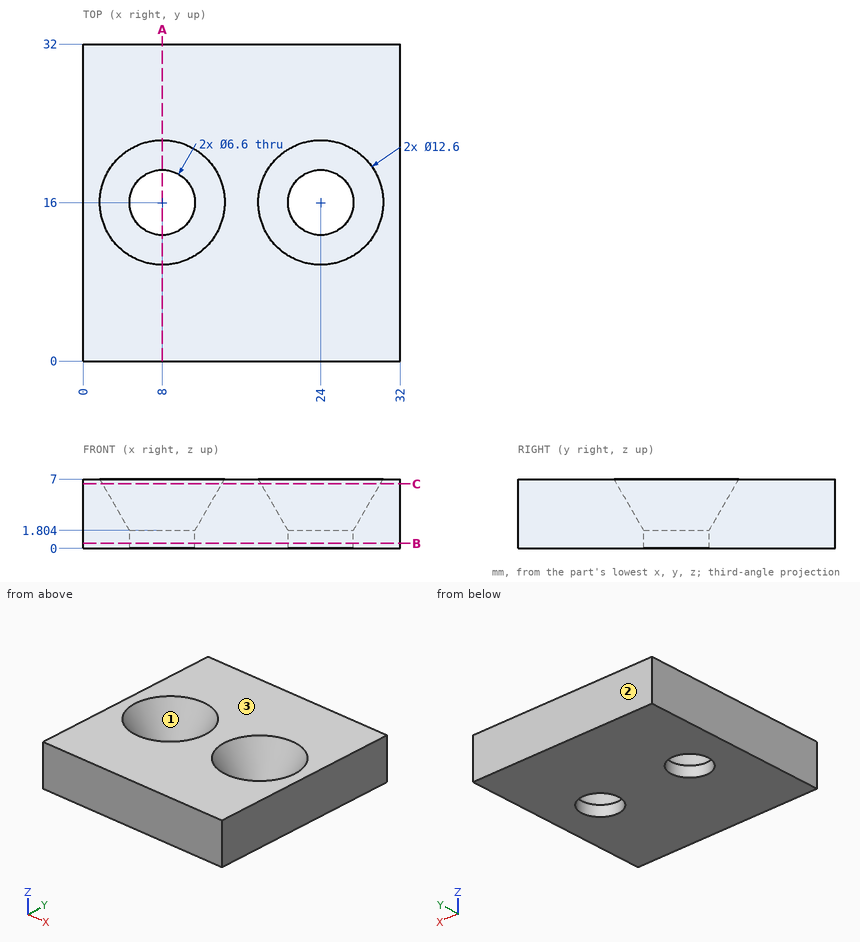
Study the drawing (mm; zero at the part's minimum x, y, z) and answer. Round coordinates to 2 decimals unless told otherwise and drop trailing zeros. Write each loop counter-clockwise with the first axis right and the second up, starting at its lowest first coordinate (ties: lowest second). Pieces come first, ordered by that corner, then holes.
1) A cutting plane is placed at A-A on x = 8. Determine the outline of the cut face in (y, z), and give its area (3 significant figures).
2) Consider probe 1 along X at (y, z) = (16, 0.85); probe 2 along Y at (x, z) = (24, 0.8); probe 3 along X at (y, z) = (21, 5.5). Determine where each line is inside the solid, lowest interval first.
3) Determine the mould class of the marked faces 1, 2 and 3 for opening direction Y: pulls with the +Y half, pulls with the -Y half, needs draft (parallel to the pull), parting line crosses it, or undercut.
4) A cutting plane is placed at C-C on z = 6.5. Determine the outline of the cut face in (x, y), and give its area (3 significant figures).
5) A cutting plane is placed at B-B on z = 0.5. Determine the outline of the cut face in (x, y), and give its area (3 significant figures).
6) Flat-ended cylindrical pins translate along their axes: P1, Ø10.5, axis at x = 8, y = 16, coming from the +Z side; P2, Ø5.5, axis at x = 24, y = 16, coming from the -Z side. Find the tip coordinate at first contact, or state that the pin passes through.
Entries:
1. outline: (0, 0) - (12.7, 0) - (12.7, 1.8) - (9.7, 7) - (0, 7) - close; (19.3, 0) - (32, 0) - (32, 7) - (22.3, 7) - (19.3, 1.8) - close
1. area: 162 mm2
2. probe 1: x = 0 to 4.7, 11.3 to 20.7, 27.3 to 32
2. probe 2: y = 0 to 12.7, 19.3 to 32
2. probe 3: x = 0 to 5.87, 10.13 to 21.87, 26.13 to 32
3. face 1: undercut
3. face 2: pulls with the +Y half
3. face 3: needs draft
4. outline: (0, 0) - (32, 0) - (32, 32) - (0, 32) - close; hole circle Ø12.02 at (8, 16); hole circle Ø12.02 at (24, 16)
4. area: 797 mm2
5. outline: (0, 0) - (32, 0) - (32, 32) - (0, 32) - close; hole circle Ø6.6 at (8, 16); hole circle Ø6.6 at (24, 16)
5. area: 956 mm2
6. P1: stops at z = 5.18
6. P2: passes through
